Study the drawing (mm; zero at the part's minimum x, y, z) and answer. Round coordinates to 2 decimals unless told otherwise and drop trailing zeros. Write each loop counter-clockwise with the first axis right and the second up, starting at its lowest first coordinate (ties: lowest second). Pieces come first, ordered by that corner, then holes. Notation, with made-up numbers: (80, 73.5) -> (114, 73.5) arc R21 ccw to (114, 90.5) -> close; hole circle Ø1 at (-21.75, 59.25). An arc over 180 degrees is marked (long way). Return JSON: item names as keys, results as strings.
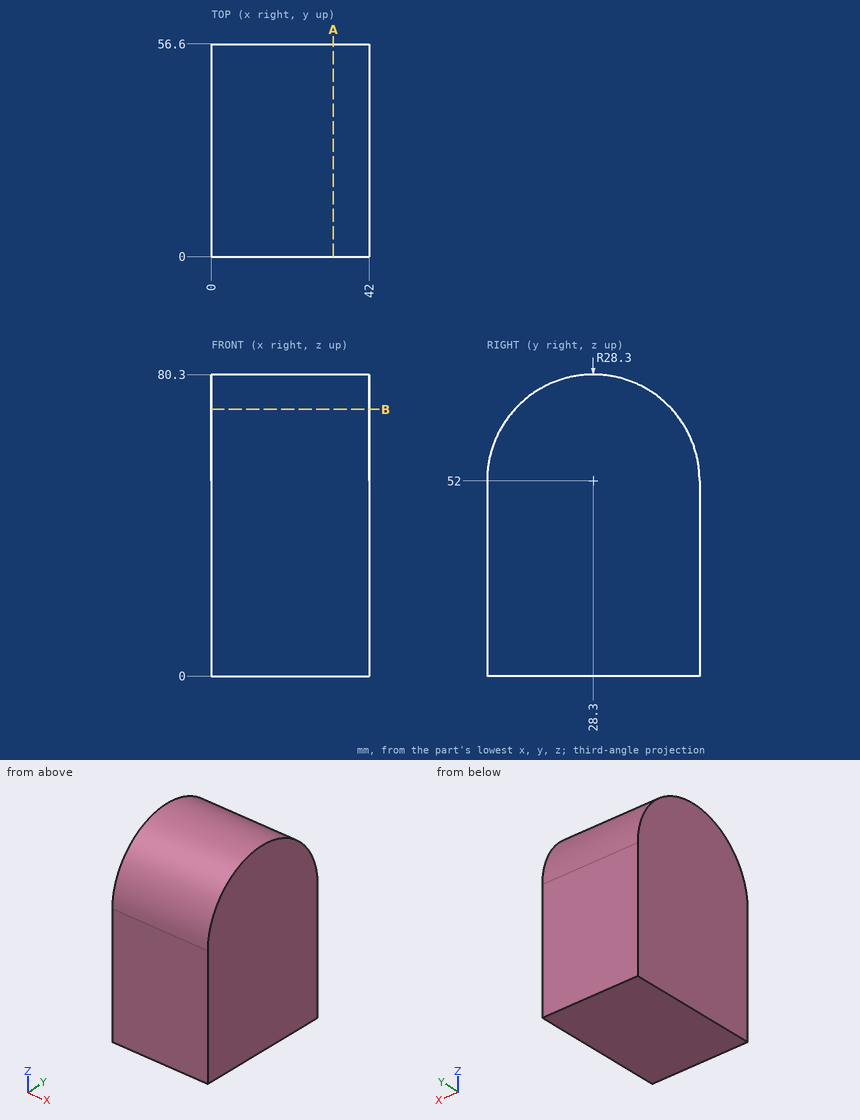
Item 1: Section A-A (x = 32.5) is taken. Give the vertices of the cut face in (y, z), then the cut area to 3 significant figures.
Worked answers:
{"outline": "(0, 0) -> (56.6, 0) -> (56.6, 52) arc R28.3 ccw to (0, 52) -> close", "area": "4,200 mm2"}
Item 2: Straight lines are drawn through the part: L1, parallel to Y at x = 5, z = 52.5; L2, parallel to Z at x = 27.5, y = 6; L3, parallel to Z at x = 11, y = 12. For each, find the intervals that lie inside material, in ascending order. Write a range as [from, to].
Worked answers:
{"L1": "y = [0, 56.6]", "L2": "z = [0, 69.42]", "L3": "z = [0, 75.13]"}
Item 3: Section B-B (z = 71) is taken. Give the vertices of the cut face in (x, y), then the cut area to 3 significant figures.
Worked answers:
{"outline": "(0, 7.33) -> (42, 7.33) -> (42, 49.27) -> (0, 49.27) -> close", "area": "1,760 mm2"}
Item 4: Flat-ended cylindrical pins translate along their axes: pin 1 (8 mm diameter, centred on x = 24, z = 38.5, fed in from -Y); pin 2 (10 mm diameter, centred on x = 37.5, y = 28, fed in from +Z). Find the tip coordinate at first contact, or state that the pin passes through.
Worked answers:
{"pin 1": "stops at y = 0", "pin 2": "stops at z = 80.3"}
